Check sheet for the modelled part. Datum: model origin and axes. Units: mm. Round coordinates to 2 decimals unless told otherwise and drop trailing zeros. Write each loop counter-clockwise with the first axis right and the second up, starting at its lowest first coordinate (ties: lowest second). Pieces come first, ordered by that corner, then holes.
Item 1: Section check A-A, the plane z = -92. Record the cut outline in (x, y).
Item 2: Section check B-B, the plane x = -2.75. Record the cut outline in (y, z), plus the area to 3 significant figures.
Item 3: Section check C-C, the plane z = 57. Record the cut outline in (x, y), plus the area to 3 significant figures.
Item 4: Release check for a two-part mould opening along X. For faces 1 (the flat face through (0, 0, -103)), 2 (the cylindrical face through (-4, -3, -14)) record: pulls with the +X half, pulls with the -X half, needs draft (parallel to the pull), parting line crosses it, or undercut.
Item 5: Material ranges on line 1 along Y through (x, z) = (0.25, -59); line 2 along X through (y, z) = (0.5, -32.5); line 3 along Y through (x, z) = (1, -7), recorded low to high.
Item 6: Depth check by flat-ended pin: pin 1 (1 mm diameter, centred on y = -2.5, z = -26.5, fed in from +X); pin 2 (0.7 mm diameter, centred on x = 3.5, y = 0.5, fed in from -Z); pin 3 (3 mm diameter, centred on x = 3, z = 53, fed in from -Y). Enter the tip coordinate at first touch or a pass-through.
from build123d import *

# Parameters (mm, degrees)
SKETCH1_R                = 5
BOSS_EXTRUDE1_DEPTH      = 72
BOSS_EXTRUDE1_DEPTH_BACK = 103
CUT_EXTRUDE1_DEPTH       = 15


with BuildPart() as part:
    # Sketch1 → Boss-Extrude1 (new body, two sides)
    with BuildSketch(Plane.XY) as boss_extrude1_sk:
        Circle(SKETCH1_R)
    extrude(amount=BOSS_EXTRUDE1_DEPTH)
    extrude(boss_extrude1_sk.sketch, amount=-BOSS_EXTRUDE1_DEPTH_BACK)

    # Sketch2 → Cut-Extrude1 (cut)
    with BuildSketch(Plane(origin=(0, 0, -103), x_dir=(-1, 0, 0), z_dir=(0, 0, -1))):
        with BuildLine():
            Line((-4.855567152, -1.193091626), (-3.196182545, -1.381362864))
            Line((-3.196182545, -1.381362864), (-2.802213635, 2.090999416))
            Line((-2.802213635, 2.090999416), (-4.458066071, 2.263989158))
            ThreePointArc((-4.458066071, 2.263989158), (-4.967272173, 0.571145479), (-4.855567152, -1.193091626))
        make_face()
    extrude(amount=-CUT_EXTRUDE1_DEPTH, mode=Mode.SUBTRACT)


solid = part.part
Values found:
1. outline: (2.8, 2.09) - (4.46, 2.26) arc R5 ccw (long way) to (4.86, -1.19) - (3.2, -1.38) - close
2. outline: (-4.18, -103) - (4.18, -103) - (4.18, 72) - (-4.18, 72) - close
2. area: 1,460 mm2
3. outline: circle Ø10 at (0, 0)
3. area: 78.5 mm2
4. face 1: needs draft
4. face 2: parting line crosses it
5. line 1: y = -4.99 to 4.99
5. line 2: x = -4.97 to 4.97
5. line 3: y = -4.9 to 4.9
6. pin 1: stops at x = 4.58
6. pin 2: stops at z = -88
6. pin 3: stops at y = -4.77
